Here's the drawing with two shaded views (mm, measured from the low corner). I have some questions. A direction names the side the tool comes from. Coordinates: 2 decimals unless noted, no trailing zeros. Write each loop counter-clockwise with the first axis right and the second up, starting at its lowest first coordinate (ties: lowest second). Pieces come first, ordered by that corner, then holes. Notation, with made-up numbers: (84, 48) -> (137, 48) arc R16 ccw to (137, 74) -> close; hole circle Ø7 at (40, 13.25). An arc over 180 degrees is marked (long way). Answer in a Markdown table with one row per item. Add a question column.
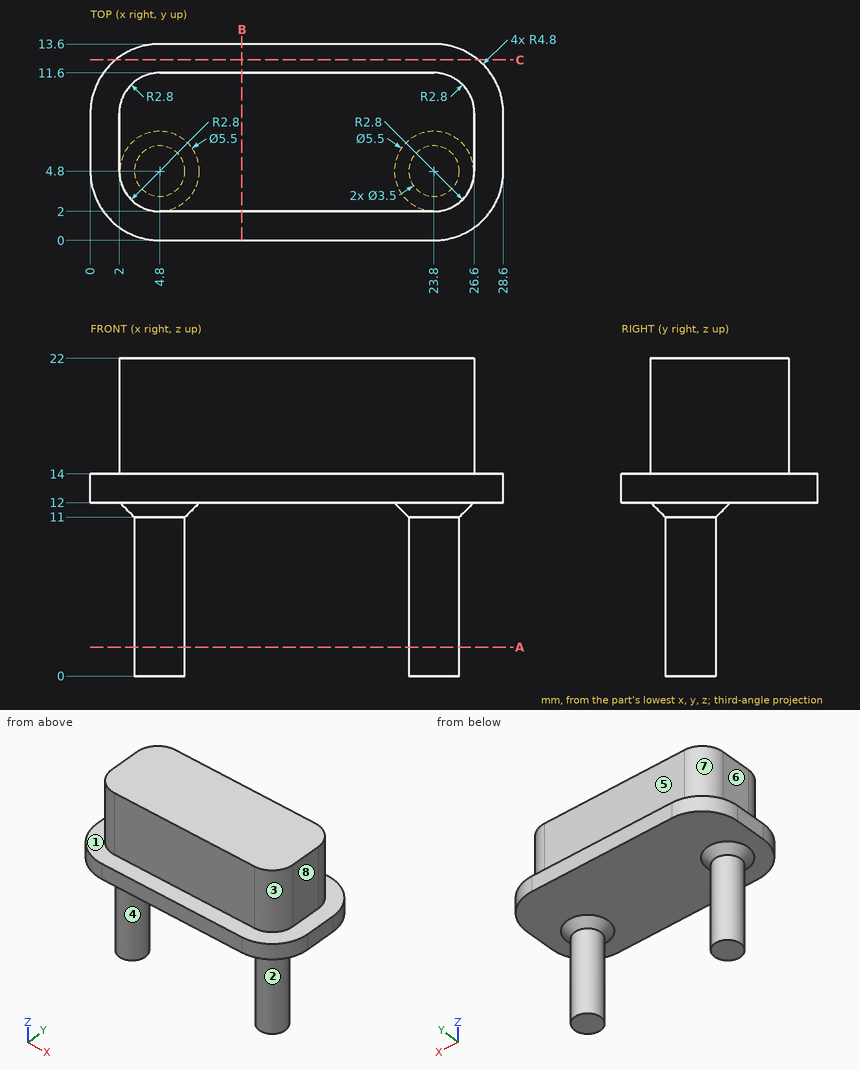
Q1. Imagine slicing it at B-B on x = 10.5. Please give me the cut outline in (y, z).
Q2. I need wall thicknesses on line 1 (Z direction, x = 17.75, y = 3.75); line 2 (Z direction, x = 4, y = 1.75); line 3 (Y direction, x = 5.25, z = 18.25). Which ranges of each line are inside material? Lowest first, please. Write a range as [from, to].
Q3. For the marked faces 4, 5, 6, 7 and 8, which set-ups out of +Z, -Z, +X, -X, +Y, -Y let a thin tool reach every point of the face, with its end or its side?
Q4. Imagine slicing it at A-A on z = 2. Please give me the cut outline in (x, y).
Q5. Imagine slicing it at C-C on y = 12.5. Please give me the cut outline in (x, z), plus the area to 3 significant figures.
Q6. If we mould it in two halves opening along X, with no side actions, what happens to the marked faces 1, 2 and 3? For each: pulls with the +X half, pulls with the -X half, needs draft (parallel to the pull), parting line crosses it, or undercut.
Q7. I'm going to push flat-ended pins straight in: P1, Ø3, axis at y = 2, z = 10, coming from the -X side; P2, Ø1.2, axis at y = 7.5, z = 19.5, coming from the -X side; P3, Ø2.5, axis at x = 15, z = 20, coming from the -Y side. Where does each tip first touch, or does it pass through?
Result sheet:
| question | item | result |
|---|---|---|
| 1 | outline | (0, 12) -> (13.6, 12) -> (13.6, 14) -> (11.6, 14) -> (11.6, 22) -> (2, 22) -> (2, 14) -> (0, 14) -> close |
| 2 | line 1 | z = [12, 22] |
| 2 | line 2 | z = [12, 14] |
| 2 | line 3 | y = [2, 11.6] |
| 3 | face 4 | -Z |
| 3 | face 5 | +Z, +X, -X, +Y |
| 3 | face 6 | +Z, -X, +Y, -Y |
| 3 | face 7 | +Z, -X, +Y |
| 3 | face 8 | +Z, +X, +Y, -Y |
| 4 | outline | circle Ø3.5 at (4.8, 4.8); circle Ø3.5 at (23.8, 4.8) |
| 5 | outline | (1.74, 12) -> (26.86, 12) -> (26.86, 14) -> (1.74, 14) -> close |
| 5 | area | 50.2 mm^2 |
| 6 | face 1 | needs draft |
| 6 | face 2 | undercut |
| 6 | face 3 | pulls with the +X half |
| 7 | P1 | stops at x = 3.63 |
| 7 | P2 | stops at x = 2 |
| 7 | P3 | stops at y = 2 |
